The model under review builds one solid part; all positions refer to its coordinate system, in mm. Face numbers are marked on the shaded views. A direction names the side the tool comes from. Coordinates: 2 decimals unless noted, no trailing zeros. Write each loop counter-clockwise with the first axis right and the second up, starting at its lowest first coordinate (ties: lowest second). Pieces come first, ordered by that corner, then holes.
```python
from build123d import *

# Parameters (mm, degrees)
BOSS_EXTRU_1_DEPTH      = 8
ESQUISSE2_R             = 17.5
ENL_V_MAT_EXTRU_1_DEPTH = 58.131427428


with BuildPart() as part:
    # Esquisse1 → Boss.-Extru.1 (new body)
    with BuildSketch(Plane.XY):
        Polygon((40, 28), (40, 32), (24, 32), (24, 40), (20, 40), (20, 32), (16, 32), (16, 40), (12, 40), (12, 32), (8, 32), (8, 40), (4, 40), (4, 32), (0, 32), (0, 40), (-8, 40), (-8, 32), (-12, 32), (-12, 40), (-16, 40), (-16, 32), (-20, 32), (-20, 40), (-24, 40), (-24, 32), (-28, 32), (-28, 40), (-32, 40), (-32, 24), (-40, 24), (-40, 20), (-32, 20), (-32, 16), (-40, 16), (-40, 12), (-32, 12), (-32, 8), (-40, 8), (-40, 4), (-32, 4), (-32, 0), (-40, 0), (-40, -8), (-32, -8), (-32, -12), (-40, -12), (-40, -16), (-32, -16), (-32, -20), (-40, -20), (-40, -24), (-32, -24), (-32, -28), (-40, -28), (-40, -32), (-24, -32), (-24, -40), (-20, -40), (-20, -32), (-16, -32), (-16, -40), (-12, -40), (-12, -32), (-8, -32), (-8, -40), (-4, -40), (-4, -32), (0, -32), (0, -40), (8, -40), (8, -32), (12, -32), (12, -40), (16, -40), (16, -32), (20, -32), (20, -40), (24, -40), (24, -32), (28, -32), (28, -40), (32, -40), (32, -24), (40, -24), (40, -20), (32, -20), (32, -16), (40, -16), (40, -12), (32, -12), (32, -8), (40, -8), (40, -4), (32, -4), (32, 0), (40, 0), (40, 8), (32, 8), (32, 12), (40, 12), (40, 16), (32, 16), (32, 20), (40, 20), (40, 24), (32, 24), (32, 28), align=None)
    extrude(amount=BOSS_EXTRU_1_DEPTH)

    # Esquisse2 → Enlèv. mat.-Extru.1 (cut, through all)
    with BuildSketch(Plane.XY):
        Circle(ESQUISSE2_R)
    extrude(amount=ENL_V_MAT_EXTRU_1_DEPTH, mode=Mode.SUBTRACT)


solid = part.part
```
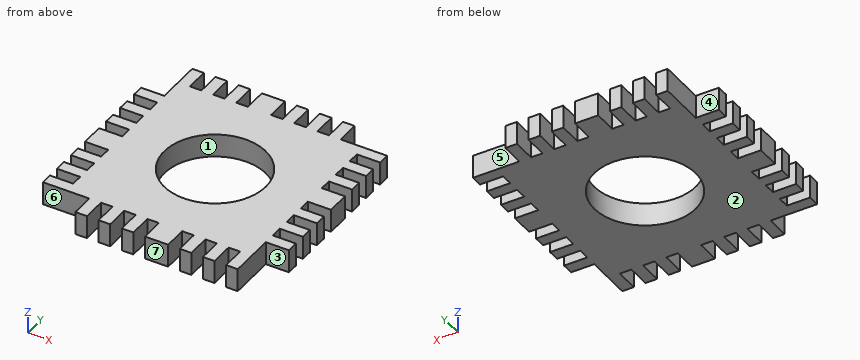
Item 1: Take a section at D-D, the plane x = -27. Write out the cut boundary in (y, z).
Solved:
outline: (-32, 0) - (32, 0) - (32, 8) - (-32, 8) - close
Item 2: For pin 1 (1.2 mm diameter, centred on x = -9, z = 2, fed in from -Y); pin 2 (4 mm diameter, centred on x = -35.5, z = 5.5, fed in from +Y); pin 3 (3 mm diameter, centred on y = -10, z = 4.5, fed in from +X), all flat-tipped, find the tip position at first contact; note any pin that passes through.
Solved:
pin 1: stops at y = -32
pin 2: stops at y = 24
pin 3: stops at x = 32
Item 3: Take a section at B-B, the plane x = -14.5. Write out the cut boundary in (y, z).
Solved:
outline: (-40, 0) - (-9.8, 0) - (-9.8, 8) - (-40, 8) - close; (9.8, 0) - (40, 0) - (40, 8) - (9.8, 8) - close
Item 4: Take a section at A-A, the plane y = 14. Write out the cut boundary in (x, z).
Solved:
outline: (-40, 0) - (-10.5, 0) - (-10.5, 8) - (-40, 8) - close; (10.5, 0) - (40, 0) - (40, 8) - (10.5, 8) - close
Item 5: To check wall thickness, follow line 1 along Y through (x, z) = (-11, 7); line 2 along Y through (x, z) = (-6, 3.75); line 3 along X through (y, z) = (-15, 0.75). State the ranges of each line that lie inside material, in increasing order.
Solved:
line 1: y = -32 to -13.61, 13.61 to 32
line 2: y = -40 to -16.44, 16.44 to 40
line 3: x = -40 to -9.01, 9.01 to 40
Item 6: Mouldability with a two-part tool opening along Y and no side actions: class the marked faces 1, 2 and 3 as pulls with the +Y half, pulls with the -Y half, needs draft (parallel to the pull), parting line crosses it, or undercut.
Solved:
face 1: undercut
face 2: needs draft
face 3: pulls with the -Y half
Item 7: Machinability: for the marked faces 4, 5, 6 and 7, which of the approach directions +Z, -Z, +X, -X, +Y, -Y give a long, thin tool a straight path to every point of the face, cutting with its end or side? Answer none if there is none.
Solved:
face 4: +Z, -Z, -X, +Y
face 5: +Z, -Z, +X, +Y
face 6: +Z, -Z, -X, -Y
face 7: +Z, -Z, +X, -X, -Y
Item 8: Take a section at C-C, the plane x = 30. Write out the cut boundary in (y, z).
Solved:
outline: (-40, 0) - (32, 0) - (32, 8) - (-40, 8) - close
